Part model, mm, in its own coordinate system. Face numbers are marked on the shaded views. A direction names the side the tool comes from. Coordinates: 2 decimals unless noted, no trailing zeros. Order: outer loops, then holes, each group sorted by start corner. A loop starts at its lowest first (then second) coordinate and runs counter-clockwise, first axis right, second up.
1) Mould opens along X. For the marked faces 4, 5, 6 and 7 say: +X half, -X half, draft (parallel to the pull), parting line (faces both ways), or undercut.
2) Pin check, flat tips, straight feed: pin 1 Ø3 at (x, z) = (-7, -11) entering from -Y; pin 2 Ø1.2 at (x, y) = (-9.5, 3) entering from +Z; pin 3 Ø1.6 at (y, z) = (3, -7.5) entering from -X. Stop position of each tip, or through.
3) Cut at C-C (z = -14). List the corners of the cut face in (x, y), and give its area (3 significant figures).
4) Cut at A-A (x = -8.5). List the corners of the cut face in (y, z).
5) Cut at B-B (y = 2.65). List the corners of the cut face in (x, z).
6) Wall check: L1, parallel to Z at x = -7.25, y = 0.7; L2, parallel to Z at x = -8.5, y = 3.7. Give the ranges that are in metal, low to high.
7) Tool access for the marked faces 1, 2 and 3: list every direction of +Z, -Z, +X, -X, +Y, -Y with a clear straight run to the whole face (end or side of a thin tool).
8) Cut at D-D (z = -2.5). List the corners of the cut face in (x, y).
Autodesk Inventor part; units mm, degrees
ref_plane "YZ Plane" through (0, 0, 0) normal (1, 0, 0) x (0, 1, 0)
ref_plane "XZ Plane" through (0, 0, 0) normal (0, 1, 0) x (-1, 0, 0)
ref_plane "XY Plane" through (0, 0, 0) normal (0, 0, 1) x (1, 0, 0)
sketch "Sketch1" plane through (0, 0, 0) normal (0, 1, 0) x (-1, 0, 0)
  line L0 (0, 0) -> (20, 0)
  line L1 (20, 0) -> (20, -20)
  line L2 (20, -20) -> (0, -20)
  line L3 (0, -20) -> (0, 0)
  dimension "d0" = 20
  dimension "d1" = 20
extrude "Extrusion1" add sketch "Sketch1" along normal blind 2
sketch "Sketch2" plane through (0, 2, 0) normal (0, 1, 0) x (1, 0, 0)
  line L0 (0, 20) -> (-20, 20)
  line L1 (-20, 20) -> (-20, 0)
  line L2 (-20, 0) -> (0, 0)
  line L3 (0, 0) -> (0, 20)
  line L4 (-18, 2) -> (-18, 18)
  line L5 (-18, 18) -> (-2, 18)
  line L6 (-2, 18) -> (-2, 2)
  line L7 (-2, 2) -> (-18, 2)
  line L8 (-16, 16) -> (-16, 4)
  line L9 (-16, 4) -> (-4, 4)
  line L10 (-4, 4) -> (-4, 16)
  line L11 (-4, 16) -> (-16, 16)
  dimension "d4" = 2
  dimension "d5" = 2
extrude "Extrusion2" add sketch "Sketch2" along normal blind 2 contours L4 L5 L6 L7
extrude "Extrusion3" cut sketch "Sketch2" against normal blind 10 contours L11 L10 L9 L8
properties part number "latticeChamberCapv4"
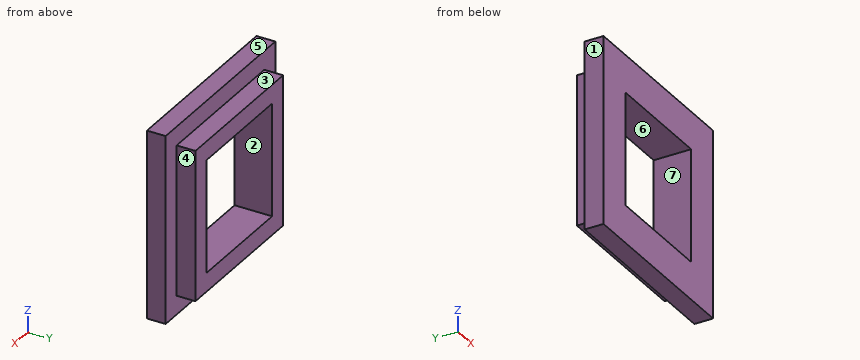
Geometry check:
1. face 4: +X half
1. face 5: draft
1. face 6: undercut
1. face 7: undercut
2. pin 1: passes through
2. pin 2: stops at z = -2
2. pin 3: stops at x = -18
3. outline: (-20, 0) - (-16, 0) - (-16, 4) - (-18, 4) - (-18, 2) - (-20, 2) - close; (-4, 0) - (0, 0) - (0, 2) - (-2, 2) - (-2, 4) - (-4, 4) - close
3. area: 24.0 mm2
4. outline: (0, -20) - (2, -20) - (2, -18) - (4, -18) - (4, -16) - (0, -16) - close; (0, -4) - (4, -4) - (4, -2) - (2, -2) - (2, 0) - (0, 0) - close
5. outline: (-18, -18) - (-2, -18) - (-2, -2) - (-18, -2) - close; hole (-16, -16) - (-4, -16) - (-4, -4) - (-16, -4) - close
6. L1: z = -20 to -16, -4 to 0
6. L2: z = -18 to -16, -4 to -2
7. face 1: +Z, -Z, -X, +Y, -Y
7. face 2: +Y, -Y
7. face 3: +Z, +X, -X, +Y
8. outline: (-20, 0) - (0, 0) - (0, 2) - (-2, 2) - (-2, 4) - (-18, 4) - (-18, 2) - (-20, 2) - close
